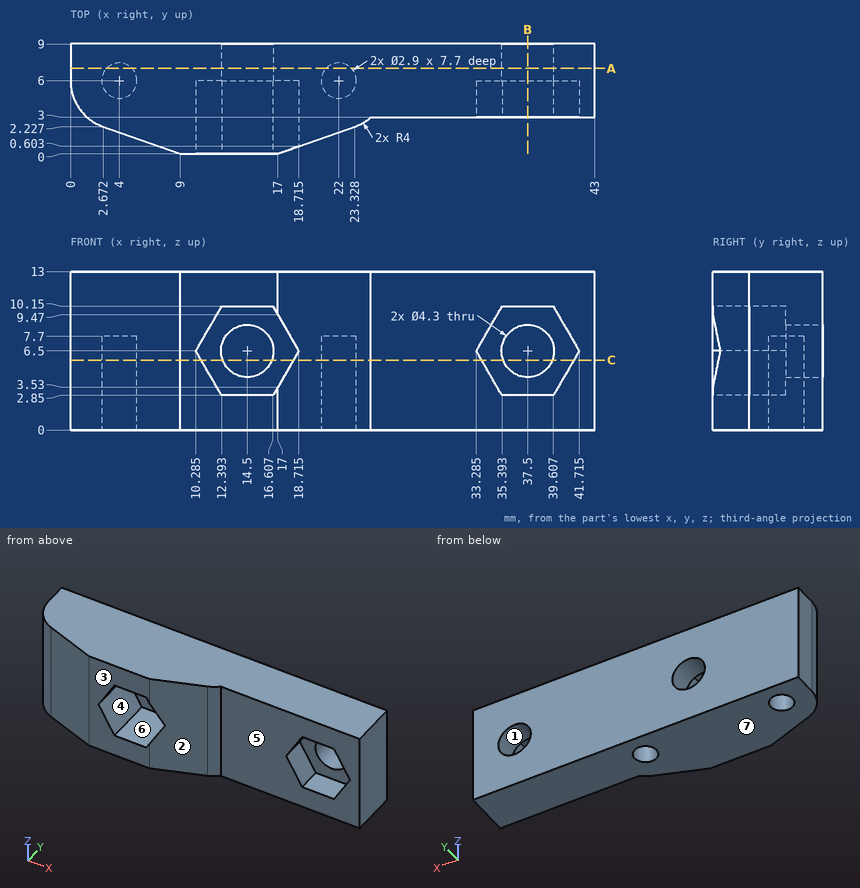
The figure shows three views and two pictorial views of one solid part (mm, origin at its lowest corner). Answer the questions. A direction names the side the tool comes from. Round coordinates to 2 decimals unless told otherwise and drop trailing zeros. Write each loop counter-clockwise with the first axis right and the second up, starting at its lowest first coordinate (ties: lowest second). Pieces come first, ordered by that corner, then holes. Notation, with made-up numbers: (72, 49.5) -> (104, 49.5) arc R12 ccw to (104, 63.5) -> close; hole circle Ø1 at (52, 73). An arc over 180 degrees is marked (long way). Answer as a JSON object with one key per item and string values. Group by question number.
Q1. Section A-A (y = 7) is taken. Write down the section's boundary in (x, z).
Q2. Each of these flat-tipped pins is pushed along its axis until it touches: pin 1 Ø4 at (x, z) = (35.5, 8) entering from -Y; pin 2 Ø0.9 at (x, y) = (22, 6.5) entering from -Z; pin 3 Ø3 at (y, z) = (2, 4) entering from -X. Where does it stop, or does it pass through?
Q3. Which of the six approach directions +Z, -Z, +X, -X, +Y, -Y give full straight-line access (tool end or side, diameter ignored) to the marked faces 5, 6 and 7?
Q4. Section C-C (z = 5.75) is taken. Count the separate pieces of the cut face and the enclosed holes in it, plus the area to 3 significant figures.
Q5. Section B-B (x = 37.5) is taken. Write down the section's boundary in (y, z), plus the area to 3 significant figures.
Q6. Determine the mould class of the marked faces 1, 2, 3 and 4 for opening direction X: pulls with the +X half, pulls with the -X half, needs draft (parallel to the pull), parting line crosses it, or undercut.
Q7. Straight lines are drawn through the part: line 1 along Z through (x, y) = (37.5, 7.3); line 2 along Z through (x, y) = (13.5, 3.5); line 3 along X through (y, z) = (5.75, 4). For each, find the intervals that lie inside material, in ascending order.
Check values:
{
 "1": {"outline": "(0, 0) -> (2.95, 0) -> (2.95, 7.7) -> (5.05, 7.7) -> (5.05, 0) -> (20.95, 0) -> (20.95, 7.7) -> (23.05, 7.7) -> (23.05, 0) -> (43, 0) -> (43, 13) -> (0, 13) -> close; hole circle Ø4.3 at (14.5, 6.5); hole circle Ø4.3 at (37.5, 6.5)"},
 "2": {"pin 1": "y = 3", "pin 2": "z = 7.7", "pin 3": "x = 0.88"},
 "3": {"face 5": "+Z, -Z, +X, -Y", "face 6": "-Y", "face 7": "-Z, +X, -X, +Y, -Y"},
 "4": {"separate pieces": "3", "enclosed holes": "2", "area": "201 mm^2"},
 "5": {"outline": "(3, 0) -> (9, 0) -> (9, 4.35) -> (6, 4.35) -> (6, 2.85) -> (3, 2.85) -> close; (3, 10.15) -> (6, 10.15) -> (6, 8.65) -> (9, 8.65) -> (9, 13) -> (3, 13) -> close", "area": "43.2 mm^2"},
 "6": {"face 1": "undercut", "face 2": "pulls with the +X half", "face 3": "needs draft", "face 4": "undercut"},
 "7": {"line 1": "0 to 4.35, 8.65 to 13", "line 2": "0 to 2.85, 10.15 to 13", "line 3": "0.01 to 2.57, 5.43 to 11.73, 17.27 to 20.57, 23.43 to 34.73, 40.27 to 43"}
}
